Design review of the part built by this model. Coordinates are the model's own, in mm. Face numbers are marked on the shaded views. Round coordinates to 2 decimals unless told otherwise and drop trailing zeros. Order: outer loops, then holes, each group sorted by start corner. A loop starts at its lowest first (then second) coordinate and runs counter-clockwise, first axis right, second up.
from build123d import *

# Parameters (mm, degrees)
SKETCH1_R           = 5
BOSS_EXTRUDE1_DEPTH = 3
SKETCH2_R           = 3.6
BOSS_EXTRUDE2_DEPTH = 3
SKETCH3_R           = 2.6
CUT_EXTRUDE1_DEPTH  = 7


with BuildPart() as part:
    # Sketch1 → Boss-Extrude1 (new body)
    with BuildSketch(Plane(origin=(0, 0, 0), x_dir=(1, 0, 0), z_dir=(0, 1, 0))):
        Circle(SKETCH1_R)
    extrude(amount=BOSS_EXTRUDE1_DEPTH)

    # Sketch2 → Boss-Extrude2 (add)
    with BuildSketch(Plane(origin=(0, 3, 0), x_dir=(1, 0, 0), z_dir=(0, 1, 0))):
        Circle(SKETCH2_R)
    extrude(amount=BOSS_EXTRUDE2_DEPTH)

    # Sketch3 → Cut-Extrude1 (cut, through all)
    with BuildSketch(Plane(origin=(0, 0, 0), x_dir=(1, 0, 0), z_dir=(0, 1, 0))):
        Circle(SKETCH3_R)
    extrude(amount=CUT_EXTRUDE1_DEPTH, mode=Mode.SUBTRACT)


solid = part.part
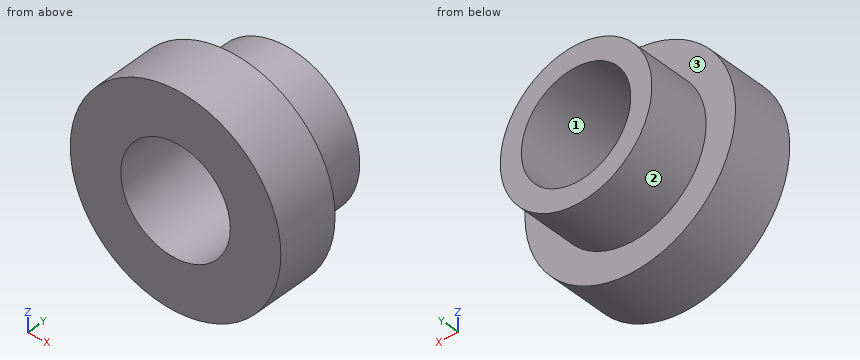
1) The part is to be moulded in two halves that separate along Z. For the marked faces 1, 2 and 3, say which applies: released by +Z, released by -Z, zero draft, split by the parting line, or undercut.
Results:
face 1: undercut
face 2: split by the parting line
face 3: zero draft
2) To check wall thickness, follow line 1 along X through (y, z) = (4.4, 0); line 2 along X through (y, z) = (2.4, 0); line 3 along Y through (x, z) = (3.5, 1.75). State the ranges of each line that lie inside material, in increasing order.
Results:
line 1: x = -3.6 to -2.6, 2.6 to 3.6
line 2: x = -5 to -2.6, 2.6 to 5
line 3: y = 0 to 3
3) Take a section at B-B on z = 0. Give the boundary of the cut face in (x, y), plus the area to 3 significant figures.
Results:
outline: (-5, 0) - (-2.6, 0) - (-2.6, 6) - (-3.6, 6) - (-3.6, 3) - (-5, 3) - close; (2.6, 0) - (5, 0) - (5, 3) - (3.6, 3) - (3.6, 6) - (2.6, 6) - close
area: 20.4 mm2
4) Take a section at A-A on x = 0. Give the boundary of the cut face in (y, z).
Results:
outline: (0, -5) - (3, -5) - (3, -3.6) - (6, -3.6) - (6, -2.6) - (0, -2.6) - close; (0, 2.6) - (6, 2.6) - (6, 3.6) - (3, 3.6) - (3, 5) - (0, 5) - close
5) Clearance check with flat-ended pins moving along their axes: P1, Ø1, axis at y = 1, z = -3.5, coming from the -X side; P2, Ø2, axis at x = 1.5, y = 2.5, coming from the -Z side; P3, Ø3, axis at x = 2.5, y = 3, coming from the -Z side. State where each tip first meets the part, or that it passes through.
Results:
P1: stops at x = -4
P2: stops at z = -4.97
P3: stops at z = -4.9
6) Take a section at C-C on y = 3.6. Give the boundary of the cut face in (x, z).
Results:
outline: circle Ø7.2 at (0, 0); hole circle Ø5.2 at (0, 0)
7) Take a section at D-D on z = 3.25. Give the boundary of the cut face in (x, y).
Results:
outline: (-3.8, 0) - (3.8, 0) - (3.8, 3) - (1.55, 3) - (1.55, 6) - (-1.55, 6) - (-1.55, 3) - (-3.8, 3) - close
